```python
from build123d import *

# Parameters (mm, degrees)
SKETCH_1_W                       = 33.2
SKETCH_1_H                       = 42.5
SM_BASE_FLANGE_1_DEPTH           = 1.5
SM_EDGE_FLANGE_1_STRIP_W         = 7.4732
SM_EDGE_FLANGE_1_STRIP_H         = 1.5
SM_EDGE_FLANGE_1_STRIP_CUT_DEPTH = 42.5
SM_EDGE_FLANGE_1_DEPTH           = 42.5
SKETCH_9_R                       = 1.25
CUT_EXTRUDE_1_DEPTH              = 10
SKETCH_10_R                      = 2.25
CUT_EXTRUDE_2_DEPTH              = 10
FILLET_1_R                       = 3


# Sheet-metal steps are written as plain solids
with BuildPart() as part:
    # Sketch 1 → 基体-法兰1 (new body)
    with BuildSketch(Plane.XY):
        Rectangle(SKETCH_1_W, SKETCH_1_H)
    extrude(amount=-SM_BASE_FLANGE_1_DEPTH)

    # 边线-法兰1 strip (across the edge) → 边线-法兰1 strip cut (cut)
    with BuildSketch(Plane(origin=(-16.6, 21.25, 0), x_dir=(1, 0, 0), z_dir=(0, -1, 0))):
        with Locations((-1.5, -0.75)):
            Rectangle(SM_EDGE_FLANGE_1_STRIP_W, SM_EDGE_FLANGE_1_STRIP_H)
    extrude(amount=SM_EDGE_FLANGE_1_STRIP_CUT_DEPTH, mode=Mode.SUBTRACT)

    # 边线-法兰1 section (across the edge) → 边线-法兰1 (add)
    with BuildSketch(Plane(origin=(-16.6, 21.25, 0), x_dir=(1, 0, 0), z_dir=(0, -1, 0))):
        with BuildLine():
            Line((0, 0.7366), (0, 10.5))
            Line((0, 10.5), (1.5, 10.5))
            Line((1.5, 10.5), (1.5, 0.7366))
            ThreePointArc((1.5, 0.7366), (1.715745145, 0.215745145), (2.2366, 0))
            Line((2.2366, 0), (2.2366, -1.5))
            ThreePointArc((2.2366, -1.5), (0.655084973, -0.844915027), (0, 0.7366))
        make_face()
    extrude(amount=SM_EDGE_FLANGE_1_DEPTH)

    # 草图9 → 切除-拉伸1 (cut)
    with BuildSketch(Plane.XY):
        with Locations((6.4, 14)):
            Circle(SKETCH_9_R)
        with Locations((-5.6, 14)):
            Circle(SKETCH_9_R)
        with Locations((6.4, -10)):
            Circle(SKETCH_9_R)
        with Locations((-5.6, -10)):
            Circle(SKETCH_9_R)
    cut_extrude_1 = extrude(amount=-CUT_EXTRUDE_1_DEPTH, mode=Mode.SUBTRACT)

    # 草图10 → 切除-拉伸2 (cut)
    with BuildSketch(Plane(origin=(-15.1, 0, 0), x_dir=(0, 0, -1), z_dir=(1, 0, 0))):
        with Locations((-6.5, 12.5)):
            Circle(SKETCH_10_R)
        with Locations((-6.5, -12.5)):
            Circle(SKETCH_10_R)
    extrude(amount=-CUT_EXTRUDE_2_DEPTH, mode=Mode.SUBTRACT)

    # 镜向1: 切除-拉伸1 across plane
    add(cut_extrude_1.mirror(Plane.ZX), mode=Mode.SUBTRACT)

    # 圆角1
    fillet_1_edges = [part.edges().sort_by_distance(p)[0] for p in [
        (-15.85, 21.25, 10.5),
        (-15.85, -21.25, 10.5),
        (16.6, 21.25, -0.75),
        (16.6, -21.25, -0.75),
    ]]
    fillet(fillet_1_edges, radius=FILLET_1_R)


solid = part.part
```
Input: part model. Units: mm. Frame: model coordinates. A direction names the side the tool comes from. Coordinates: 2 decimals unless noted, no trailing zeros. Write each loop counter-clockwise with the first axis right and the second up, starting at its lowest first coordinate (ties: lowest second). Pieces come first, ordered by that corner, then holes. Notation, with made-up numbers: (28, -38.75) -> (84, -38.75) arc R13 ccw to (84, -19.75) -> close; hole circle Ø7 at (71, 52). An arc over 180 degrees is marked (long way). Write each question's results on one line, items separated by ' | '.
Item 1: Section query C-C on y = 14. Return loops of the section in (x, z).
Conclusion:
outline: (-16.6, 0.74) arc R2.24 ccw to (-14.36, -1.5) -> (-6.85, -1.5) -> (-6.85, 0) -> (-14.36, 0) arc R0.74 cw to (-15.1, 0.74) -> (-15.1, 4.82) -> (-16.6, 4.82) -> close; (-16.6, 8.18) -> (-15.1, 8.18) -> (-15.1, 10.5) -> (-16.6, 10.5) -> close; (-4.35, -1.5) -> (5.15, -1.5) -> (5.15, 0) -> (-4.35, 0) -> close; (7.65, -1.5) -> (16.6, -1.5) -> (16.6, 0) -> (7.65, 0) -> close
Item 2: Material intervals for probe 1 along Y at (x, z) = (6.4, -0.6); probe 2 along Y at (x, z) = (-15.7, 6.5); probe 3 along Z at (x, y) = (5, -16), sorted ascending.
Conclusion:
probe 1: y = -21.25 to -15.25, -12.75 to -11.25, -8.75 to 8.75, 11.25 to 12.75, 15.25 to 21.25 | probe 2: y = -21.25 to -14.75, -10.25 to 10.25, 14.75 to 21.25 | probe 3: z = -1.5 to 0
Item 3: Section query D-D on y = -8. Return loops of the section in (x, z).
Conclusion:
outline: (-16.6, 0.74) arc R2.24 ccw to (-14.36, -1.5) -> (16.6, -1.5) -> (16.6, 0) -> (-14.36, 0) arc R0.74 cw to (-15.1, 0.74) -> (-15.1, 10.5) -> (-16.6, 10.5) -> close
Item 4: Section query B-B on x = 6.4. Return loops of the section in (y, z), plus the area to 4 significant figures.
Conclusion:
outline: (-21.25, -1.5) -> (-15.25, -1.5) -> (-15.25, 0) -> (-21.25, 0) -> close; (-12.75, -1.5) -> (-11.25, -1.5) -> (-11.25, 0) -> (-12.75, 0) -> close; (-8.75, -1.5) -> (8.75, -1.5) -> (8.75, 0) -> (-8.75, 0) -> close; (11.25, -1.5) -> (12.75, -1.5) -> (12.75, 0) -> (11.25, 0) -> close; (15.25, -1.5) -> (21.25, -1.5) -> (21.25, 0) -> (15.25, 0) -> close | area: 48.75 mm^2
Item 5: Set-up query: faces 1 (the cylindrical face through (-15.93, 0.3, -0.86)), 2 (the flat face through (-15.1, 0, 6)). Return all of +Z, -Z, +X, -X, +Y, -Y with unobstructed straight access to the full face (end or side cutting, diameter ignored); none if empty.
Conclusion:
face 1: -Z, -X, +Y, -Y | face 2: +Z, +X, +Y, -Y
Item 6: Mould query, pull axis X, two halves, no side actions, for faces 3 (the cylindrical face through (15.7, -20.39, -0.76)), 4 (the cylindrical face through (6.24, 15.24, -0.74)), 5 (the flat face through (1, 0, 0)). Classes: +X half, -X half, draft (parallel to the pull), parting line (faces both ways), or undercut.
Conclusion:
face 3: +X half | face 4: undercut | face 5: draft
Item 7: Pin query (flat end, axial travel): pin 1 Ø7 at (y, z) = (12.5, 6.5) entering from +X; pin 2 Ø3 at (x, y) = (-5.6, -14) entering from +Z. Return the tip coordinate at first contact, or that it passes through.
Conclusion:
pin 1: stops at x = -15.1 | pin 2: stops at z = 0
Item 8: Section query A-A on z = 6.5. Return loops of the section in (x, y), plus the area to 4 significant figures.
Conclusion:
outline: (-16.6, -21.25) -> (-15.1, -21.25) -> (-15.1, -14.75) -> (-16.6, -14.75) -> close; (-16.6, -10.25) -> (-15.1, -10.25) -> (-15.1, 10.25) -> (-16.6, 10.25) -> close; (-16.6, 14.75) -> (-15.1, 14.75) -> (-15.1, 21.25) -> (-16.6, 21.25) -> close | area: 50.25 mm^2
